```python
from build123d import *

# Parameters (mm, degrees)
F1_DEPTH = 40
F2_R     = 1
F3_DEPTH = 7.851
F6_R     = 4
F8_R     = 2


with BuildPart() as f1:
    # F0 (on Top) → F1 (new body)
    with BuildSketch(Plane.XY):
        Polygon((0, 3.62576), (-3.14, 1.81288), (-3.14, -1.81288), (0, -3.62576), (3.14, -1.81288), (3.14, 1.81288), align=None)
    extrude(amount=F1_DEPTH)

    # F2 (on face) → F3 (cut, through all)
    with BuildSketch(Plane(origin=(1.57, -2.71932, 0), x_dir=(0.866025, 0.5, 0), z_dir=(0.5, -0.866025, 0))):
        with Locations((0, 35)):
            Circle(F2_R)
    extrude(amount=-F3_DEPTH, mode=Mode.SUBTRACT)

    # F7: sweep along a path in F5
    with BuildLine(Plane.XY.offset(10.5)) as f7_path:
        CenterArc((0, 0), 6.75, 0, 360)
    # F6 (on Front) → F7 (sweep, cut)
    with BuildSketch(Plane.XZ):
        with Locations((-6.75, 10.5)):
            Circle(F6_R)
    sweep(path=f7_path.line, mode=Mode.SUBTRACT)

    # F8
    f8_edges = [f1.edges().sort_by_distance(p)[0] for p in [
        (1.57, -2.71932, 40),
        (-1.57, -2.71932, 40),
        (3.14, 0, 40),
        (-1.57, 2.71932, 40),
        (-3.14, 0, 40),
        (1.57, 2.71932, 40),
    ]]
    fillet(f8_edges, radius=F8_R)


solid = f1.part
```
Build history of the part. All positions in model axes, mm. Round coordinates to 2 decimals unless told otherwise and drop trailing zeros. Order: outer loops, then holes, each group sorted by start corner. A loop starts at its lowest first (then second) coordinate and runs counter-clockwise, first axis right, second up. Notation, with made-up numbers: (37.25, -38.5) -> (75.25, -38.5) arc R29 ccw to (75.25, -18.5) -> close; hole circle Ø6 at (71, 57.25). An arc over 180 degrees is marked (long way). Answer in a Markdown table with one row per item.
1) Pin check, flat tip, straight feed: P1, Ø1, axis at x = 1.5, y = 1.5, coming from the +Z side. Stop position of the tip, or through.
Values:
| item | result |
|---|---|
| P1 | z = 39.96 |
2) Mould opens along Y. For faces 1 (the cylindrical face through (2.766, 0.025, 39.165)), 2 (the flat face through (1.55, -2.73, 4.33)), 3 (the cylindrical face through (0, 0, 36)), 4 (the cylindrical face through (-1.4, 2.38, 39.17)) say: released by +Y, released by -Y, zero draft, split by the parting line, or undercut.
Values:
| item | result |
|---|---|
| face 1 | zero draft |
| face 2 | released by -Y |
| face 3 | undercut |
| face 4 | released by +Y |
3) Band-saw the part on A-A on z = 27. Give the cut face in (x, y).
Values:
| item | result |
|---|---|
| outline | (-3.14, -1.81) -> (0, -3.63) -> (3.14, -1.81) -> (3.14, 1.81) -> (0, 3.63) -> (-3.14, 1.81) -> close |
4) Wall check: L1, parallel to Z at x = -0.5, y = 2; L2, parallel to Z at x = -1.75, y = 1.25; L3, parallel to Y at x = 1.75, z = 28. Give the ranges that are in metal, low to high.
Values:
| item | result |
|---|---|
| L1 | 0 to 34.18, 35.82 to 39.81 |
| L2 | 0 to 34.55, 35.45 to 39.83 |
| L3 | -2.62 to 2.62 |
